from build123d import *

# Parameters (mm, degrees)
F0_W     = 50.8
F0_H     = 50.8
F1_DEPTH = 50.8
F3_DEPTH = 2.54


with BuildPart() as f1:
    # F0 (on Front) → F1 (new body)
    with BuildSketch(Plane.XZ):
        with Locations((25.4, 25.4)):
            Rectangle(F0_W, F0_H)
    extrude(amount=F1_DEPTH)

    # F2 (on face) → F3 (cut)
    with BuildSketch(Plane.XZ.offset(50.8)):
        Polygon((19.194489, 39.729136), (14.504312, 44.419312), (8.097411, 42.702589), (6.380688, 36.295688), (11.070864, 31.605511), (17.477765, 33.322235), align=None)
        Polygon((44.419312, 36.295688), (42.702589, 42.702589), (36.295688, 44.419312), (31.605511, 39.729136), (33.322235, 33.322235), (39.729136, 31.605511), align=None)
        Polygon((14.504312, 6.380688), (19.194489, 11.070864), (17.477765, 17.477765), (11.070864, 19.194489), (6.380688, 14.504312), (8.097411, 8.097411), align=None)
        Polygon((33.322235, 17.477765), (31.605511, 11.070864), (36.295688, 6.380688), (42.702589, 8.097411), (44.419312, 14.504312), (39.729136, 19.194489), align=None)
    extrude(amount=-F3_DEPTH, mode=Mode.SUBTRACT)


solid = f1.part
Design review of the part built by this model. Coordinates are the model's own, in mm. A direction names the side the tool comes from. Coordinates: 2 decimals unless noted, no trailing zeros. Use a Markdown table: item, result. Add a question column.
Item 1: Machinability: for faces 4 (the flat face through (8.693, -49.548, 33.983)), 5 (the flat face through (25, -25, 0)), which of the approach directions +Z, -Z, +X, -X, +Y, -Y give a long, thin tool a straight path to every point of the face, cutting with its end or side? Answer none if there is none.
Item 2: The part is to be moulded in two halves that separate along X. For faces 1 (the flat face through (50.8, -25, 25)), 2 (the flat face through (25, -50.8, 26)), 3 (the flat face through (43.573, -49.548, 39.454)), say which applies: +X half, -X half, draft (parallel to the pull), parting line (faces both ways), or undercut.
Item 3: Wall thickness on L1, parallel to Y at x = 39.5, z = 7.5: over which ranges is the line inside the solid? List them lowest first. Write a range as from..to.
Numbers:
| question | item | result |
|---|---|---|
| 1 | face 4 | -Y |
| 1 | face 5 | -Z, +X, -X, +Y, -Y |
| 2 | face 1 | +X half |
| 2 | face 2 | draft |
| 2 | face 3 | undercut |
| 3 | L1 | y = -48.26..0 |
